Geometry: see drawing. Coordinates: mm, zero at the bounding-box minimum. Give positions to 0.01 mm unless a question says otherwise; leave off trailing zeros. Order: outer loops, then holes, each group sorted by start corner. A loop starts at its lowest first (then second) coordinate and runs counter-clockwise, first axis right, second up. Notation, with made-up numbers: (57, 89.5) -> (90, 89.5) arc R21 cw to (90, 118.5) -> close; hole circle Ø10 at (36, -11.5). An arc over 180 degrees is marked (long way). Use one line per item in the form item = value. Start each with the question number.
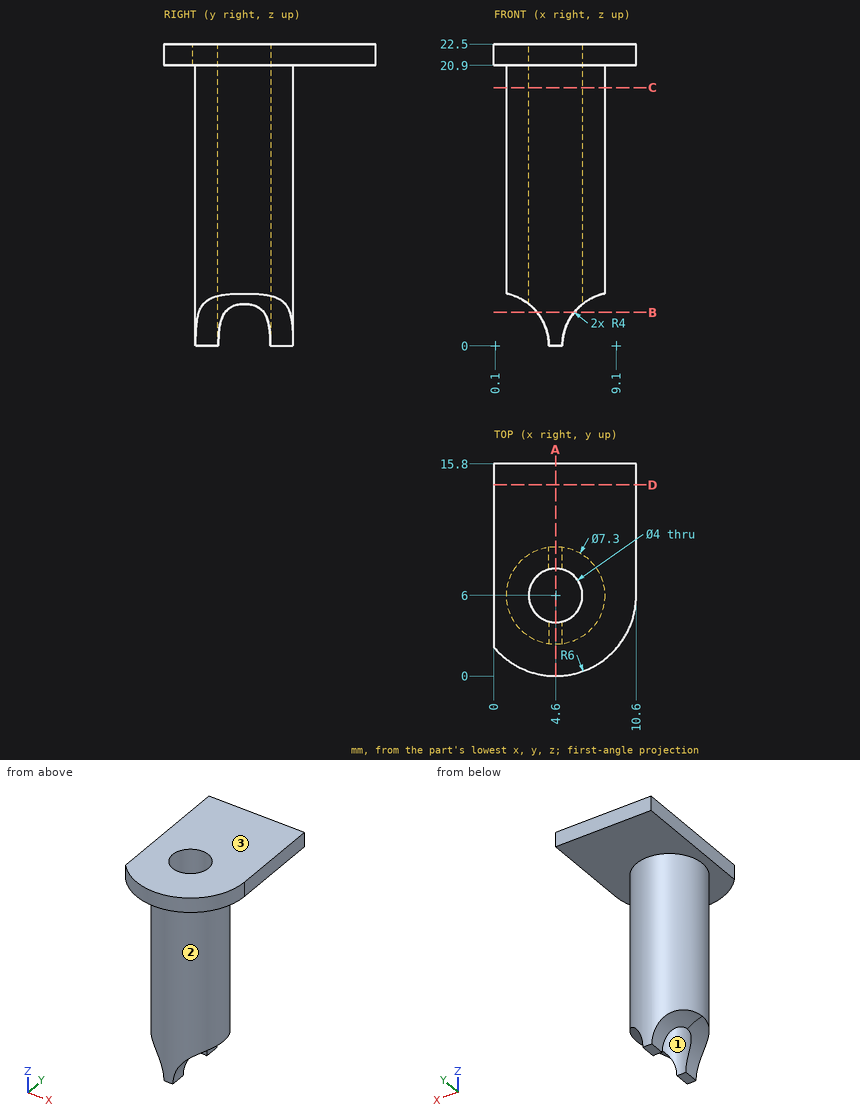
1) Pin query (flat end, axial travel): pin 1 (3 mm diameter, centred on x = 5, z = 5, fed in from -Y); pin 2 (1 mm diameter, centred on x = 5, z = 16, fed in from +Y); pin 3 (2 mm diameter, centred on x = 7.5, z = 15.5, fed in from +Y). Return the tip coordinate at first contact, or that it passes through.
2) Material intervals for probe 1 along Y at (x, z) = (4.6, 16); probe 2 along X at (y, z) = (6, 16); probe 3 along Z at (x, y) = (1.25, 13.5), sorted ascending.
3) Draft query along X for the marked faces 1, 2 and 3. Return one class per face: +X half, -X half, draft (parallel to the pull), parting line (faces both ways), or undercut.
4) Cut plane D-D, the plane y = 14.25. Return the cut outline in (x, z).
5) Cut plane A-A, the plane x = 4.6. Return the cut outline in (y, z).
6) Cut plane C-C, the plane z = 19.25. Return the cut outline in (x, y), plus the area to 3 significant figures.
7) Cut plane B-B, the plane z = 2.5. Return the cut outline in (x, y).
Output values:
q1.pin_1 = 2.35
q1.pin_2 = 9.65
q1.pin_3 = 9.12
q2.probe_1 = 2.35 to 4, 8 to 9.65
q2.probe_2 = 0.95 to 2.6, 6.6 to 8.25
q2.probe_3 = 20.9 to 22.5
q3.face_1 = undercut
q3.face_2 = parting line
q3.face_3 = draft
q4.outline = (0, 20.9) -> (10.6, 20.9) -> (10.6, 22.5) -> (0, 22.5) -> close
q5.outline = (0, 20.9) -> (2.35, 20.9) -> (2.35, 0) -> (4, 0) -> (4, 22.5) -> (0, 22.5) -> close; (8, 0) -> (9.65, 0) -> (9.65, 20.9) -> (15.8, 20.9) -> (15.8, 22.5) -> (8, 22.5) -> close
q6.outline = circle Ø7.3 at (4.6, 6); hole circle Ø4 at (4.6, 6)
q6.area = 29.3 mm^2
q7.outline = (3.22, 2.62) arc R3.65 ccw to (5.98, 2.62) -> (5.98, 4.55) arc R2 cw to (3.22, 4.55) -> close; (3.22, 7.45) arc R2 cw to (5.98, 7.45) -> (5.98, 9.38) arc R3.65 ccw to (3.22, 9.38) -> close
